```python
from build123d import *

# Parameters (mm, degrees)
BOSS_EXTRUDE1_START = 4.7625
SKETCH3_R           = 7.14375
SKETCH3_R_2         = 3.9878
BOSS_EXTRUDE1_DEPTH = 1.5875
BOSS_EXTRUDE2_START = 3.175
SKETCH4_R           = 5.588
SKETCH4_R_2         = 3.9878
BOSS_EXTRUDE2_DEPTH = 7.9375
CHAMFER1_SIZE       = 0.119634


with BuildPart() as part:
    # Sketch3 → Boss-Extrude1 (new body)
    with BuildSketch(Plane.XY.offset(BOSS_EXTRUDE1_START)):
        Circle(SKETCH3_R)
        Circle(SKETCH3_R_2, mode=Mode.SUBTRACT)
    extrude(amount=-BOSS_EXTRUDE1_DEPTH)

    # Sketch4 → Boss-Extrude2 (add)
    with BuildSketch(Plane.XY.offset(BOSS_EXTRUDE2_START)):
        Circle(SKETCH4_R)
        Circle(SKETCH4_R_2, mode=Mode.SUBTRACT)
    extrude(amount=-BOSS_EXTRUDE2_DEPTH)

    # Chamfer1
    chamfer1_edges = [part.edges().sort_by_distance(p)[0] for p in [
        (-3.9878, 0, -4.7625),
        (-5.588, 0, 3.175),
        (-7.14375, 0, 4.7625),
        (-7.14375, 0, 3.175),
        (-3.9878, 0, 4.7625),
        (-5.588, 0, -4.7625),
    ]]
    chamfer(chamfer1_edges, length=CHAMFER1_SIZE)


solid = part.part
```
The listing builds one solid part. Answer for the finished solid, in the listing's coordinates (mm). A direction names the side the tool comes from. Round coordinates to 2 decimals unless told otherwise and drop trailing zeros. Loops run counter-clockwise (first coordinate to the right, second up) from the corner with the lowest first, then second, coordinate; pieces in that order, holes last.
1) For a pull along X with two mould halves and no side action, classify faces 3 (the face through (-7.137, 0.314, 3.978)), 4 (the face through (0, 6, 3.175)), 5 (the face through (3.804, 1.198, 0.065)) as released by +X, released by -X, zero draft, split by the parting line, or undercut.
Outcome:
face 3: split by the parting line
face 4: zero draft
face 5: undercut
2) A cutting plane is placed at D-D on z = 3.5. Determine the outline of the cut face in (x, y), plus the area to 3 significant figures.
Outcome:
outline: circle Ø14.29 at (0, 0); hole circle Ø7.98 at (0, 0)
area: 110 mm2
3) Consider line 1 (Y direction, x = 0, z = 2.5); line 2 (Z direction, x = -3.25, y = -5) (1 decimal); line 3 (Y direction, x = -1.25, z = 2.25). Determine where each line is inside the solid, lowest interval first.
Outcome:
line 1: y = -5.59 to -3.99, 3.99 to 5.59
line 2: z = 3.2 to 4.8
line 3: y = -5.45 to -3.79, 3.79 to 5.45
4) Given P1, Ø2, axis at x = 5, z = -1, coming from the -Y side; P2, Ø4, axis at y = -0.5, z = -3.5, coming from the -X side; P3, Ø5, axis at y = 4, z = 2, coming from the -X side, each flat-ended and moving along its own axis, determine where each tip first touches the part or whether it passes through.
Outcome:
P1: stops at y = -3.9
P2: stops at x = -5.59
P3: stops at x = -6.9
5) A cutting plane is placed at C-C on z = -0.25. Determine the outline of the cut face in (x, y).
Outcome:
outline: circle Ø11.18 at (0, 0); hole circle Ø7.98 at (0, 0)
6) For faces 1 (the face through (2, 4, -4.762)), 2 (the face through (-4.434, -3.4, -0.74)), determine the directions among +Z, -Z, +X, -X, +Y, -Y from which every point of the face is accessible in a straight line to the end or side of a thin tool.
Outcome:
face 1: -Z, +X, -X, +Y, -Y
face 2: -Z
